The model under review builds one solid part; all positions refer to its coordinate system, in mm. A direction names the side the tool comes from. Give positions to 0.01 mm unless a question says otherwise; leave off trailing zeros. Order: outer loops, then holes, each group sorted by start corner. A loop starts at its lowest first (then second) coordinate and runs counter-clockwise, first axis right, second up.
```python
from build123d import *

# Parameters (mm, degrees)
SKETCH1_R                = 12.7
BOSS_EXTRUDE1_DEPTH      = 15.367
BOSS_EXTRUDE1_DEPTH_BACK = 15.367
SKETCH4_W                = 25.4
SKETCH4_H                = 30.734
CUT_EXTRUDE2_DEPTH       = 3.71145
SKETCH5_W                = 14.2875
SKETCH5_H                = 16.637
CUT_EXTRUDE3_DEPTH       = 13.7
CUT_EXTRUDE3_DEPTH_BACK  = 13.7
CUT_EXTRUDE4_DEPTH       = 20.9771001
SKETCH7_R                = 4.7625
CUT_EXTRUDE5_DEPTH       = 31.7340001
SKETCH9_R                = 17.852773039
SKETCH9_R_2              = 9.9822
CUT_EXTRUDE6_DEPTH       = 4.572
SKETCH10_R               = 6.477
CUT_EXTRUDE7_DEPTH       = 24.257
SKETCH11_R               = 3.175
CUT_EXTRUDE8_DEPTH       = 20.9771001
SKETCH12_R               = 0.79375
CUT_EXTRUDE9_DEPTH       = 1.0000001
CUT_EXTRUDE9_DEPTH_BACK  = 20.9771001
SKETCH15_R               = 4.7625
CUT_EXTRUDE12_DEPTH      = 4.445
SKETCH16_R               = 1.5875
CUT_EXTRUDE13_DEPTH      = 4.445


with BuildPart() as part:
    # Sketch1 → Boss-Extrude1 (new body, two sides)
    with BuildSketch(Plane(origin=(0, 0, 0), x_dir=(1, 0, 0), z_dir=(0, 1, 0))) as boss_extrude1_sk:
        Circle(SKETCH1_R)
    extrude(amount=BOSS_EXTRUDE1_DEPTH)
    extrude(boss_extrude1_sk.sketch, amount=-BOSS_EXTRUDE1_DEPTH_BACK)

    # Sketch4 → Cut-Extrude2 (cut, through all)
    with BuildSketch(Plane.XY.offset(9.98855)):
        Rectangle(SKETCH4_W, SKETCH4_H)
    cut_extrude2 = extrude(amount=CUT_EXTRUDE2_DEPTH, mode=Mode.SUBTRACT)

    # Mirror2: Cut-Extrude2 across plane
    add(cut_extrude2.mirror(Plane.XY), mode=Mode.SUBTRACT)

    # Sketch5 → Cut-Extrude3 (cut, two sides)
    with BuildSketch(Plane(origin=(0, 0, 0), x_dir=(0, 0, -1), z_dir=(1, 0, 0))) as cut_extrude3_sk:
        with Locations((0, 7.0485)):
            Rectangle(SKETCH5_W, SKETCH5_H)
        with BuildLine():
            Line((7.14375, -1.27), (-7.14375, -1.27))
            ThreePointArc((-7.14375, -1.27), (0, -8.41375), (7.14375, -1.27))
        make_face()
    extrude(amount=CUT_EXTRUDE3_DEPTH, mode=Mode.SUBTRACT)
    extrude(cut_extrude3_sk.sketch, amount=-CUT_EXTRUDE3_DEPTH_BACK, mode=Mode.SUBTRACT)

    # Sketch6 → Cut-Extrude4 (cut, through all)
    with BuildSketch(Plane.XY.offset(9.98855)):
        with BuildLine():
            ThreePointArc((7.843396515, 11.847950137), (9.813665145, 8.601547837), (10.50036, 4.86664))
            Line((10.50036, 4.86664), (14.849727138, 4.86664))
            ThreePointArc((14.849727138, 4.86664), (0, 19.716367138), (-14.849727138, 4.86664))
            Line((-14.849727138, 4.86664), (-10.50036, 4.86664))
            ThreePointArc((-10.50036, 4.86664), (-9.813665145, 8.601547837), (-7.843396515, 11.847950137))
            Line((-7.843396515, 11.847950137), (-7.843396515, 15.367))
            Line((-7.843396515, 15.367), (0, 15.367))
            Line((0, 15.367), (7.843396515, 15.367))
            Line((7.843396515, 15.367), (7.843396515, 11.847950137))
        make_face()
        with BuildLine():
            ThreePointArc((-7.843396515, 11.847950137), (-4.298330514, 14.446927831), (0, 15.367))
            Line((0, 15.367), (-7.843396515, 15.367))
            Line((-7.843396515, 15.367), (-7.843396515, 11.847950137))
        make_face()
        with BuildLine():
            ThreePointArc((0, 15.367), (4.298330514, 14.446927831), (7.843396515, 11.847950137))
            Line((7.843396515, 11.847950137), (7.843396515, 15.367))
            Line((7.843396515, 15.367), (0, 15.367))
        make_face()
    extrude(amount=-CUT_EXTRUDE4_DEPTH, mode=Mode.SUBTRACT)

    # Sketch7 → Cut-Extrude5 (cut, through all)
    with BuildSketch(Plane.XZ.offset(15.367)):
        Circle(SKETCH7_R)
    extrude(amount=-CUT_EXTRUDE5_DEPTH, mode=Mode.SUBTRACT)

    # Sketch9 → Cut-Extrude6 (cut)
    with BuildSketch(Plane.XZ.offset(15.367)):
        Circle(SKETCH9_R)
        Circle(SKETCH9_R_2, mode=Mode.SUBTRACT)
    extrude(amount=-CUT_EXTRUDE6_DEPTH, mode=Mode.SUBTRACT)

    # Sketch10 → Cut-Extrude7 (cut)
    with BuildSketch(Plane(origin=(0, 15.367, 0), x_dir=(1, 0, 0), z_dir=(0, 1, 0))):
        Circle(SKETCH10_R)
    extrude(amount=-CUT_EXTRUDE7_DEPTH, mode=Mode.SUBTRACT)

    # Sketch11 → Cut-Extrude8 (cut, through all)
    with BuildSketch(Plane.XY.offset(9.98855)):
        with Locations((0, 7.747)):
            Circle(SKETCH11_R)
    extrude(amount=-CUT_EXTRUDE8_DEPTH, mode=Mode.SUBTRACT)

    # Sketch12 → Cut-Extrude9 (cut, two sides)
    with BuildSketch(Plane(origin=(0, 0, -9.98855), x_dir=(-1, 0, 0), z_dir=(0, 0, -1))) as cut_extrude9_sk:
        with Locations((5.081146515, -4.445)):
            Circle(SKETCH12_R)
        with Locations((-5.081146515, -4.445)):
            Circle(SKETCH12_R)
    extrude(amount=CUT_EXTRUDE9_DEPTH, mode=Mode.SUBTRACT)
    extrude(cut_extrude9_sk.sketch, amount=-CUT_EXTRUDE9_DEPTH_BACK, mode=Mode.SUBTRACT)

    # Sketch15 → Cut-Extrude12 (cut)
    with BuildSketch(Plane.XZ.offset(15.367)):
        with BuildLine():
            ThreePointArc((8.001, 0), (-5.572105758, 5.741745241), (-0.239879494, -7.997403255))
            Line((-0.239879494, -7.997403255), (7.597144444, -2.509860017))
            ThreePointArc((7.597144444, -2.509860017), (7.899390916, -1.271072049), (8.001, 0))
        make_face()
        Circle(SKETCH15_R, mode=Mode.SUBTRACT)
    extrude(amount=-CUT_EXTRUDE12_DEPTH, mode=Mode.SUBTRACT)

    # Sketch16 → Cut-Extrude13 (cut)
    with BuildSketch(Plane.XZ.offset(15.367)):
        with Locations((-0.217023554, -7.235403255)):
            Circle(SKETCH16_R)
        with Locations((6.873606877, -2.270825729)):
            Circle(SKETCH16_R)
    extrude(amount=-CUT_EXTRUDE13_DEPTH, mode=Mode.SUBTRACT)


solid = part.part
```
Item 1: Take a section at D-D (x = 5.25). Give the boundary of the cut face in (y, z) (1 decimal), and give its area (3 significant figures).
Values found:
outline: (-15.4, -8.5) - (-10.8, -8.5) - (-10.8, -10) - (-5.2, -10) - (-5.2, -6) arc R7.1 cw to (-7.3, -3.8) - (-8.9, -3.8) - (-8.9, 3.8) - (-7.3, 3.8) arc R7.1 cw to (-5.2, 6) - (-5.2, 10) - (-10.8, 10) - (-10.8, 8.5) - (-15.4, 8.5) - (-15.4, 6) - (-10.9, 6) - (-10.9, -4.2) - (-15.4, -4.2) - close; (-3.7, -10) - (14, -10) - (14, -7.1) - (-1.3, -7.1) arc R7.1 cw to (-3.7, -6.7) - close; (-3.7, 6.7) arc R7.1 cw to (-1.3, 7.1) - (14, 7.1) - (14, 10) - (-3.7, 10) - close
area: 212 mm2
Item 2: Take a section at B-B (x = -3.75). Give the boundary of the cut face in (y, z) (1 decimal), and give its area (3 significant figures).
Values found:
outline: (-15.4, -9.3) - (-10.8, -9.3) - (-10.8, -10) - (14.7, -10) - (14.7, -7.1) - (-1.3, -7.1) arc R7.1 cw to (-6.1, -5.3) - (-8.9, -5.3) - (-8.9, -2.9) - (-10.9, -2.9) - (-10.9, -7.1) - (-15.4, -7.1) - close; (-15.4, 7.1) - (-10.9, 7.1) - (-10.9, 2.9) - (-8.9, 2.9) - (-8.9, 5.3) - (-6.1, 5.3) arc R7.1 cw to (-1.3, 7.1) - (14.7, 7.1) - (14.7, 10) - (-10.8, 10) - (-10.8, 9.3) - (-15.4, 9.3) - close
area: 198 mm2
Item 3: For line 1 (Z direction, x = 5.5, y = 2); line 2 (Y direction, x = 0, z = 8.8); line 3 (Y direction, x = 0, z = -8.5), list the stretches that pass through material, from the lowest coordinate up.
Values found:
line 1: z = -9.99 to -7.14, 7.14 to 9.99
line 2: y = -15.37 to 4.57, 10.92 to 15.37
line 3: y = -10.92 to 4.57, 10.92 to 15.37
Item 4: Take a section at A-A (z = 3.5). Give the boundary of the cut face in (x, y) (1 decimal), and give its area (3 significant figures).
Values found:
outline: (-12.2, -10.8) - (-9.3, -10.8) - (-9.3, -15.4) - (-7.2, -15.4) - (-7.2, -10.9) - (-3.2, -10.9) - (-3.2, -8.9) - (-5.4, -8.9) - (-5.4, -7.5) - (-12.2, -7.5) - close; (3.2, -10.9) - (7.2, -10.9) - (7.2, -15.4) - (9.3, -15.4) - (9.3, -10.8) - (12.2, -10.8) - (12.2, -7.5) - (5.4, -7.5) - (5.4, -8.9) - (3.2, -8.9) - close
area: 73.7 mm2
Item 5: Clearance check with flat-ended pins moving along their axes: pin 1 Ø8.5 at (x, y) = (2.5, 8.5) entering from -Z; pin 2 Ø1.3 at (x, y) = (5.08, -4.44) entering from +Z; pin 3 Ø11.5 at (x, z) = (0, 0) entering from +Y; pin 4 Ø10.5 at (x, z) = (-2.5, -1) entering from +Y. State where each tip first meets the part, or that it passes through.
Values found:
pin 1: stops at z = -9.99
pin 2: passes through
pin 3: stops at y = -8.89
pin 4: stops at y = -4.73
Item 6: For faces 5 (the flat face through (-2, 5, 7.144)), 6 (the flat face through (-8, -10.795, -7)), 7 (the cylindrical face through (-4.91, -5.22, -7.99)), list the 3-axis set-ups (+Z, -Z, +X, -X, +Y, -Y) from which the entire face can be reached by the end or side of a thin tool; tool diameter is ignored.
Values found:
face 5: +X, -X, +Y
face 6: -Y
face 7: +Z, -Z
Item 7: Draft analysis for pull direction Y (two halves, no side actions). For faces 1 (the flat face through (0, -8.89, -5)), 2 (the flat face through (0, 2, -9.989)), 3 (the flat face through (4.4, -15.367, -5.2)), 4 (the cylindrical face through (-0.688, 4.648, 8.586)), state which applies: released by +Y, released by -Y, zero draft, split by the parting line, or undercut.
Values found:
face 1: released by +Y
face 2: zero draft
face 3: released by -Y
face 4: undercut
Item 8: Take a section at C-C (y = -10). Give the boundary of the cut face in (x, z) (1 decimal), and give its area (3 significant figures).
Values found:
outline: (-7.8, -10) - (7.8, -10) arc R12.7 ccw to (7.8, 10) - (-7.8, 10) arc R12.7 ccw to start; hole circle Ø9.5 at (0, 0)
area: 377 mm2
